Can you work these out from the model? Positions are in its coordinate system, mm. A direction names the side the tool comes from. Give positions to 0.01 mm unless a question says otherwise; leave off trailing zeros. Order: outer loops, then holes, each group sorted by start corner. A loop starts at its lowest first (then second) coordinate and runs counter-clockwise, first axis right, second up. Notation, with made-up numbers: (-34, 16) -> (-22, 16) arc R11 ccw to (-22, 22) -> close; hole circle Ø7 at (-28.75, -14.5). An arc over 180 degrees is marked (long way). Answer as CSV lines item,"result".
```python
from build123d import *

# Parameters (mm, degrees)
SKETCH1_W           = 28
SKETCH1_H           = 12
SKETCH1_R           = 1.45
BOSS_EXTRUDE1_DEPTH = 3
SKETCH2_W           = 58
SKETCH2_H           = 3
BOSS_EXTRUDE2_DEPTH = 10
SKETCH3_R           = 1.75
CUT_EXTRUDE1_DEPTH  = 12


with BuildPart() as part:
    # Sketch1 → Boss-Extrude1 (new body)
    with BuildSketch(Plane(origin=(0, 0, 0), x_dir=(1, 0, 0), z_dir=(0, 1, 0))):
        with Locations((14, -6)):
            Rectangle(SKETCH1_W, SKETCH1_H)
        with Locations(Location((6.5, -5, 0), (0, 0, 270))):
            Circle(SKETCH1_R, mode=Mode.SUBTRACT)
        with Locations(Location((21.5, -5, 0), (0, 0, 270))):
            Circle(SKETCH1_R, mode=Mode.SUBTRACT)
    extrude(amount=BOSS_EXTRUDE1_DEPTH)

    # Sketch2 → Boss-Extrude2 (add)
    with BuildSketch(Plane(origin=(0, 3, 0), x_dir=(1, 0, 0), z_dir=(0, 1, 0))):
        with Locations((14, 1.5)):
            Rectangle(SKETCH2_W, SKETCH2_H)
    extrude(amount=-BOSS_EXTRUDE2_DEPTH)

    # Sketch3 → Cut-Extrude1 (cut)
    with BuildSketch(Plane(origin=(0, 0, -3), x_dir=(-1, 0, 0), z_dir=(0, 0, -1))):
        with Locations((9, -2.359486917)):
            Circle(SKETCH3_R)
        with Locations((-36.998595295, -2)):
            Circle(SKETCH3_R)
        with Locations((2, -2)):
            Circle(SKETCH3_R)
        with Locations((-30, -2)):
            Circle(SKETCH3_R)
    extrude(amount=-CUT_EXTRUDE1_DEPTH, mode=Mode.SUBTRACT)


solid = part.part
```
Item 1: For pin 1 (2 mm diameter, centred on x = -9, y = -2.36, fed in from +Z); pin 2 (1.5 mm diameter, centred on y = 1, z = 2, fed in from -X); pin 3 (4 mm diameter, centred on x = 6.5, z = 5, fed in from -Y); pin 4 (2 mm diameter, centred on x = -2.5, y = 1, fed in from +Z), each with a flat end and sliding along its axis, tell me the tip position at first contact or that it passes through.
Numbers:
pin 1,"passes through"
pin 2,"stops at x = 0"
pin 3,"stops at y = 0"
pin 4,"stops at z = 0"
Item 2: Please list where these lines run through material, in increasing order: line 1 along X through (y, z) = (0.25, 5); line 2 along X through (y, z) = (-1.25, -2.5); line 3 along X through (y, z) = (1.5, 4.25).
Numbers:
line 1,"x = 0 to 5.05, 7.95 to 20.05, 22.95 to 28"
line 2,"x = -15 to -10.35, -7.65 to -3.58, -0.42 to 28.42, 31.58 to 35.42, 38.58 to 43"
line 3,"x = 0 to 5.26, 7.74 to 20.26, 22.74 to 28"
Item 3: We'd pull the mould along X, two halves only. Please class faces 6 (the cylindrical face through (-9.81, -3.91, -1.52)), 7 (the cylindrical face through (-3.617, -2.67, -1.521)), 8 (the flat face through (14, -2, -3)), 9 (the flat face through (43, -2, -1)): released by +X, released by -X, zero draft, split by the parting line, or undercut.
Numbers:
face 6,"undercut"
face 7,"undercut"
face 8,"zero draft"
face 9,"released by +X"
Item 4: Imagine slicing it at D-D, the plane x = 30. Please give me the cut outline in (y, z).
Numbers:
outline,"(-7, -3) -> (-3.75, -3) -> (-3.75, 0) -> (-7, 0) -> close; (-0.25, -3) -> (3, -3) -> (3, 0) -> (-0.25, 0) -> close"
Item 5: Imagine slicing it at A-A, the plane x = 6.5. Please give me the cut outline in (y, z).
Numbers:
outline,"(-7, -3) -> (3, -3) -> (3, 3.55) -> (0, 3.55) -> (0, 0) -> (-7, 0) -> close; (0, 6.45) -> (3, 6.45) -> (3, 12) -> (0, 12) -> close"
Item 6: Imagine slicing it at B-B, the plane z = 4.5. Please give me the cut outline in (x, y).
Numbers:
outline,"(0, 0) -> (5.14, 0) -> (5.14, 3) -> (0, 3) -> close; (7.86, 0) -> (20.14, 0) -> (20.14, 3) -> (7.86, 3) -> close; (22.86, 0) -> (28, 0) -> (28, 3) -> (22.86, 3) -> close"
Item 7: Imagine slicing it at C-C, the plane y = 0.75. Please give me the cut outline in (x, z).
Numbers:
outline,"(-15, -3) -> (43, -3) -> (43, 0) -> (28, 0) -> (28, 12) -> (0, 12) -> (0, 0) -> (-15, 0) -> close; hole circle Ø2.9 at (6.5, 5); hole circle Ø2.9 at (21.5, 5)"
Item 8: For faces 1 (the flat face through (0, 1, 6)), 2 (the flat face through (14, -7, -2)), 3 (the cylindrical face through (35.38, -2.67, -1.52)), 4 (the flat face through (14, 0, 6)), 5 (the flat face through (28, 1, 6)), which set-ups out of +Z, -Z, +X, -X, +Y, -Y let a thin tool reach every point of the face, with its end or its side?
Numbers:
face 1,"+Z, -X, +Y, -Y"
face 2,"+Z, -Z, +X, -X, -Y"
face 3,"+Z, -Z"
face 4,"+Z, +X, -X, -Y"
face 5,"+Z, +X, +Y, -Y"
